```python
from build123d import *

# Parameters (mm, degrees)
F1_DEPTH = 6.35
F2_R     = 2.5
F3_DEPTH = 1.5
F4_R     = 0.5
F5_DEPTH = 25.4


with BuildPart() as f1:
    # F0 (on Front) → F1 (new body)
    with BuildSketch(Plane.XZ):
        with BuildLine():
            ThreePointArc((0, 1.635), (1.1561195872, 1.1561195872), (1.635, 0))
            Line((1.635, 0), (5.25, 0))
            ThreePointArc((5.25, 0), (3.7123106012, 3.7123106012), (0, 5.25))
            Line((0, 5.25), (0, 1.635))
        make_face()
        with BuildLine():
            Line((5.25, 0), (1.635, 0))
            ThreePointArc((1.635, 0), (-1.1561195872, -1.1561195872), (0, 1.635))
            Line((0, 1.635), (0, 5.25))
            ThreePointArc((0, 5.25), (-3.7123106012, -3.7123106012), (5.25, 0))
        make_face()
        with BuildLine():
            ThreePointArc((0, 5.25), (3.7123106012, 3.7123106012), (5.25, 0))
            Line((5.25, 0), (34.25, 0))
            ThreePointArc((34.25, 0), (35.7876893988, 3.7123106012), (39.5, 5.25))
            Line((39.5, 5.25), (39.5, 19.75))
            ThreePointArc((39.5, 19.75), (35.7876893988, 21.2876893988), (34.25, 25))
            Line((34.25, 25), (5.25, 25))
            ThreePointArc((5.25, 25), (3.7123106012, 21.2876893988), (0, 19.75))
            Line((0, 19.75), (0, 5.25))
        make_face()
        with BuildLine():
            ThreePointArc((39.5, 5.25), (35.7876893988, 3.7123106012), (34.25, 0))
            Line((34.25, 0), (37.865, 0))
            ThreePointArc((37.865, 0), (38.3438804128, 1.1561195872), (39.5, 1.635))
            Line((39.5, 1.635), (39.5, 5.25))
        make_face()
        with BuildLine():
            Line((37.865, 0), (34.25, 0))
            ThreePointArc((34.25, 0), (39.5, -5.25), (44.75, 0))
            ThreePointArc((44.75, 0), (43.2123106012, 3.7123106012), (39.5, 5.25))
            Line((39.5, 5.25), (39.5, 1.635))
            ThreePointArc((39.5, 1.635), (40.6561195872, 1.1561195872), (41.135, 0))
            ThreePointArc((41.135, 0), (39.5, -1.635), (37.865, 0))
        make_face()
        with BuildLine():
            ThreePointArc((5.25, 25), (-3.7123106012, 28.7123106012), (0, 19.75))
            Line((0, 19.75), (0, 23.365))
            ThreePointArc((0, 23.365), (-1.1561195872, 26.1561195872), (1.635, 25))
            Line((1.635, 25), (5.25, 25))
        make_face()
        with BuildLine():
            Line((0, 23.365), (0, 19.75))
            ThreePointArc((0, 19.75), (3.7123106012, 21.2876893988), (5.25, 25))
            Line((5.25, 25), (1.635, 25))
            ThreePointArc((1.635, 25), (1.1561195872, 23.8438804128), (0, 23.365))
        make_face()
        with BuildLine():
            ThreePointArc((34.25, 25), (35.7876893988, 21.2876893988), (39.5, 19.75))
            Line((39.5, 19.75), (39.5, 23.365))
            ThreePointArc((39.5, 23.365), (38.3438804128, 23.8438804128), (37.865, 25))
            Line((37.865, 25), (34.25, 25))
        make_face()
        with BuildLine():
            Line((39.5, 23.365), (39.5, 19.75))
            ThreePointArc((39.5, 19.75), (43.2123106012, 21.2876893988), (44.75, 25))
            ThreePointArc((44.75, 25), (39.5, 30.25), (34.25, 25))
            Line((34.25, 25), (37.865, 25))
            ThreePointArc((37.865, 25), (39.5, 26.635), (41.135, 25))
            ThreePointArc((41.135, 25), (40.6561195872, 23.8438804128), (39.5, 23.365))
        make_face()
    extrude(amount=F1_DEPTH)

    # F2 (on face) → F3 (cut)
    with BuildSketch(Plane.XZ.offset(6.35)):
        with Locations((0, 25)):
            Circle(F2_R)
        with Locations((39.5, 25)):
            Circle(F2_R)
        with Locations((39.5, 0)):
            Circle(F2_R)
        Circle(F2_R)
    extrude(amount=-F3_DEPTH, mode=Mode.SUBTRACT)

    # F4 (on face) → F5 (cut)
    with BuildSketch(Plane(origin=(0, 0, 0), x_dir=(-1, 0, 0), z_dir=(0, 1, 0))):
        with Locations((-32.95, 12.5)):
            Circle(F4_R)
        with BuildLine():
            ThreePointArc((-6.05, 12.5), (-6.55, 13), (-7.05, 12.5))
            ThreePointArc((-7.05, 12.5), (-6.55, 12), (-6.05, 12.5))
        make_face()
    extrude(amount=-F5_DEPTH, mode=Mode.SUBTRACT)


solid = f1.part
```
Geometry check sheet. Reference: the model listing, model coordinates, mm. A direction names the side the tool comes from. Give positions to 0.01 mm unless a question says otherwise; leave off trailing zeros. Loops run counter-clockwise (first coordinate to the right, second up) from the corner with the lowest first, then second, coordinate; pieces in that order, holes last. Notation, with made-up numbers: M 38,-19 L 84,-19 A23 cw 84,-10 Z; hole C 20.25,89 d10. An arc over 180 degrees is marked long. Answer as CSV lines item,"result".
Item 1: Material ranges on line 1 (Z direction, x = 6.55, y = -3.75); line 2 (Z direction, x = 40.5, y = -5.75); line 3 (X direction, y = -0.75, z = 1), recorded low to high.
Values:
line 1,"z = 0 to 12, 13 to 25"
line 2,"z = -5.15 to -2.29, 2.29 to 5.15, 19.85 to 22.71, 27.29 to 30.15"
line 3,"x = -5.15 to -1.29, 1.29 to 38.21, 40.79 to 44.65"
Item 2: Release check for a two-part mould opening along Z. For faces 1 (the flat face through (19, -6.35, 13)), 2 (the cylindrical face through (32.488, -3.131, 12.308)), 3 (the flat face through (20, -3, 25)), 4 (the cylindrical face through (-0.54, -5.61, -2.44)) record: pulls with the +Z half, pulls with the -Z half, needs draft (parallel to the pull), parting line crosses it, or undercut.
Values:
face 1,"needs draft"
face 2,"undercut"
face 3,"pulls with the +Z half"
face 4,"undercut"
Item 3: Cross-section at D-D on x = 8.5. Record the cut outline in (y, z).
Values:
outline,"M -6.35,0 L 0,0 L 0,25 L -6.35,25 Z"
Item 4: Access from +Z, -Z, +X, -X, +Y, -Y to the whole of each face (thin tool, end or side, straight path). Record for faces 5 (the flat face through (1, -4.85, 23)), 6 (the flat face through (39.5, -3, 12)), 7 (the flat face through (20, -3, 0)).
Values:
face 5,"-Y"
face 6,"+X, +Y, -Y"
face 7,"-Z, +Y, -Y"
Item 5: Cross-section at B-B on y = -4.25. Record the cut outline in (x, z) (3 decimals), and give its area (3 significant figures).
Values:
outline,"M 0,5.25 A5.25 ccw long 5.25,0 L 34.25,0 A5.25 ccw long 39.5,5.25 L 39.5,19.75 A5.25 ccw long 34.25,25 L 5.25,25 A5.25 ccw long 0,19.75 Z; hole C 0,0 d3.27; hole C 0,25 d3.27; hole C 6.55,12.5 d1; hole C 32.95,12.5 d1; hole C 39.5,0 d3.27; hole C 39.5,25 d3.27"
area,"1,210 mm²"
Item 6: Depth check by flat-ended pin: P1, Ø4, axis at x = 0, z = 0, coming from the +Y side; P2, Ø1, axis at y = -4.5, z = 3, coming from the -X side; P3, Ø2.5, axis at x = 40, z = 25.5, coming from the -Y side; P4, Ø3, axis at x = 0, z = 0, coming from the -Y side. Enter the tip coordinate at first touch or a pass-through.
Values:
P1,"stops at y = 0"
P2,"stops at x = -4.62"
P3,"stops at y = -4.85"
P4,"passes through"
Item 7: Cross-section at A-A on z = 12.5. Record the cut outline in (x, y).
Values:
outline,"M 0,-6.35 L 6.05,-6.35 L 6.05,0 L 0,0 Z; M 7.05,-6.35 L 32.45,-6.35 L 32.45,0 L 7.05,0 Z; M 33.45,-6.35 L 39.5,-6.35 L 39.5,0 L 33.45,0 Z"
Item 8: Cross-section at C-C on x = 32.95. Record the cut outline in (y, z).
Values:
outline,"M -6.35,0 L 0,0 L 0,12 L -6.35,12 Z; M -6.35,13 L 0,13 L 0,25 L -6.35,25 Z"
